```python
from build123d import *

# Parameters (mm, degrees)
EXTRUDE_1_DEPTH = 52
SKETCH_2_R      = 9
EXTRUDE_2_DEPTH = 34
EXTRUDE_3_DEPTH = 22


with BuildPart() as part:
    # 스케치1 → 보스-돌출1 (new body)
    with BuildSketch(Plane.XY):
        with BuildLine():
            Line((0, 34), (108, 34))
            ThreePointArc((108, 34), (142, 0), (108, -34))
            Line((108, -34), (0, -34))
            ThreePointArc((0, -34), (-34, 0), (0, 34))
        make_face()
        with BuildLine():
            Line((0, 15), (108, 15))
            ThreePointArc((108, 15), (123, 0), (108, -15))
            Line((108, -15), (0, -15))
            ThreePointArc((0, -15), (-15, 0), (0, 15))
        make_face(mode=Mode.SUBTRACT)
    extrude(amount=EXTRUDE_1_DEPTH)

    # 스케치2 → 보스-돌출2 (add)
    with BuildSketch(Plane.XY):
        with BuildLine():
            Line((108, 34), (68, 34))
            ThreePointArc((68, 34), (78.606601718, 38.393398282), (83, 49))
            Line((83, 49), (83, 76))
            ThreePointArc((83, 76), (108, 101), (133, 76))
            Line((133, 76), (133, 23.043437244))
            ThreePointArc((133, 23.043437244), (121.647767834, 31.140623519), (108, 34))
        make_face()
        with Locations((108, 76)):
            Circle(SKETCH_2_R, mode=Mode.SUBTRACT)
    extrude(amount=EXTRUDE_2_DEPTH)

    # 스케치3 → 보스-돌출3 (add)
    with BuildSketch(Plane.XY):
        with BuildLine():
            Line((-16.891194038, 29.507415407), (95.037714778, 97.377070936))
            ThreePointArc((95.037714778, 97.377070936), (86.216323421, 88.266679857), (83, 76))
            Line((83, 76), (83, 49))
            ThreePointArc((83, 49), (78.606601718, 38.393398282), (68, 34))
            Line((68, 34), (0, 34))
            ThreePointArc((0, 34), (-8.739218391, 32.857663671), (-16.891194038, 29.507415407))
        make_face()
    extrude(amount=EXTRUDE_3_DEPTH)


solid = part.part
```
Could you check a few things on this model? Use its own coordinates, in mm. A direction names the side the tool comes from. Coordinates: 2 decimals unless noted, no trailing zeros. Write each loop counter-clockwise with the first axis right and the second up, starting at its lowest first coordinate (ties: lowest second). Pieces come first, ordered by that corner, then holes. Notation, with made-up numbers: (40.25, 73.25) -> (57.25, 73.25) arc R27 ccw to (57.25, 97.25) -> close; hole circle Ø3 at (79.5, 73). An arc over 180 degrees is marked (long way). One line per question, with ' | ' between items. Start each with the question number.
1. If we section it at D-D (x = 26): Please give me the cut outline in (y, z).
2. If we section it at C-C (z = 38): Please give me the cut outline in (x, y).
3. Please list where these lines run through material, in increasing order: line 1 along Y through (x, z) = (108, 24); line 2 along Y through (x, z) = (15.5, 31); line 3 along Y through (x, z) = (100.5, 9.5).
4. Will these pins go through, and if not, where does the flat tip stop? P1, Ø6, axis at y = 27, z = 43.5, coming from the -X side; P2, Ø6, axis at y = 68.5, z = 31, coming from the -X side; P3, Ø12, axis at y = 63, z = 6.5, coming from the -X side.
5. If we section it at A-A (y = 0): Please give me the cut outline in (x, z), and give its area (3 significant figures).
6. For faces 5 (the face through (53, 15, 26)), 6 (the face through (133, 50, 17)), 7 (the face through (78.49, 38.28, 27.92)), which set-ups out of +Z, -Z, +X, -X, +Y, -Y let a thin tool reach every point of the face, with its end or its side?
7. If we section it at B-B (z = 26.5): Please give me the cut outline in (x, y), and give its area (3 significant figures).
8. Thinking about a two-plate mould opening in X: for faces 1 (the face through (140.2, -10.92, 25.64)), 2 (the face through (116.032, 99.675, 16.762)), 3 (the face through (-15, 0, 26)), 4 (the face through (41, 34, 37)), which applies, pulls with the +X half, pulls with the -X half, needs draft (parallel to the pull), parting line crosses it, or undercut?
Return value:
1) outline: (-34, 0) -> (-15, 0) -> (-15, 52) -> (-34, 52) -> close; (15, 0) -> (55.52, 0) -> (55.52, 22) -> (34, 22) -> (34, 52) -> (15, 52) -> close
2) outline: (0, -34) -> (108, -34) arc R34 ccw to (108, 34) -> (0, 34) arc R34 ccw to start; hole (0, -15) -> (108, -15) arc R15 ccw to (108, 15) -> (0, 15) arc R15 ccw to start
3) line 1: y = -34 to -15, 15 to 67, 85 to 101 | line 2: y = -34 to -15, 15 to 34 | line 3: y = -34 to -15, 15 to 71.03, 80.97 to 99.85
4) P1: stops at x = -24.08 | P2: stops at x = 83 | P3: stops at x = 28.45
5) outline: (-34, 0) -> (-15, 0) -> (-15, 52) -> (-34, 52) -> close; (123, 0) -> (142, 0) -> (142, 52) -> (123, 52) -> close | area: 1,980 mm²
6) face 5: +Z, -Z | face 6: +Z, -Z, +X, +Y | face 7: +Z, -X, +Y
7) outline: (0, -34) -> (108, -34) arc R34 ccw to (133, 23.04) -> (133, 76) arc R25 ccw to (83, 76) -> (83, 49) arc R15 cw to (68, 34) -> (0, 34) arc R34 ccw to start; hole (0, -15) -> (108, -15) arc R15 ccw to (108, 15) -> (0, 15) arc R15 ccw to start; hole circle Ø18 at (108, 76) | area: 9,990 mm²
8) face 1: pulls with the +X half | face 2: parting line crosses it | face 3: undercut | face 4: needs draft
